Verification items for this drawing (mm, ordinates from the low corner). Round coordinates to 2 decimals unless told otherwise and drop trailing zeros. Write each loop counter-clockwise with the first axis right and the second up, starting at its lowest first coordinate (ties: lowest second). Pieces come first, ordered by that corner, then holes. Notation, with made-up numbers: (-9, -16.75) -> (50, -16.75) arc R6 ccw to (50, -9.75) -> close; hole circle Ø10 at (44, -6.75). An arc over 180 degrees is marked (long way). Put each result on its own line as item: value. Start each with the question number.
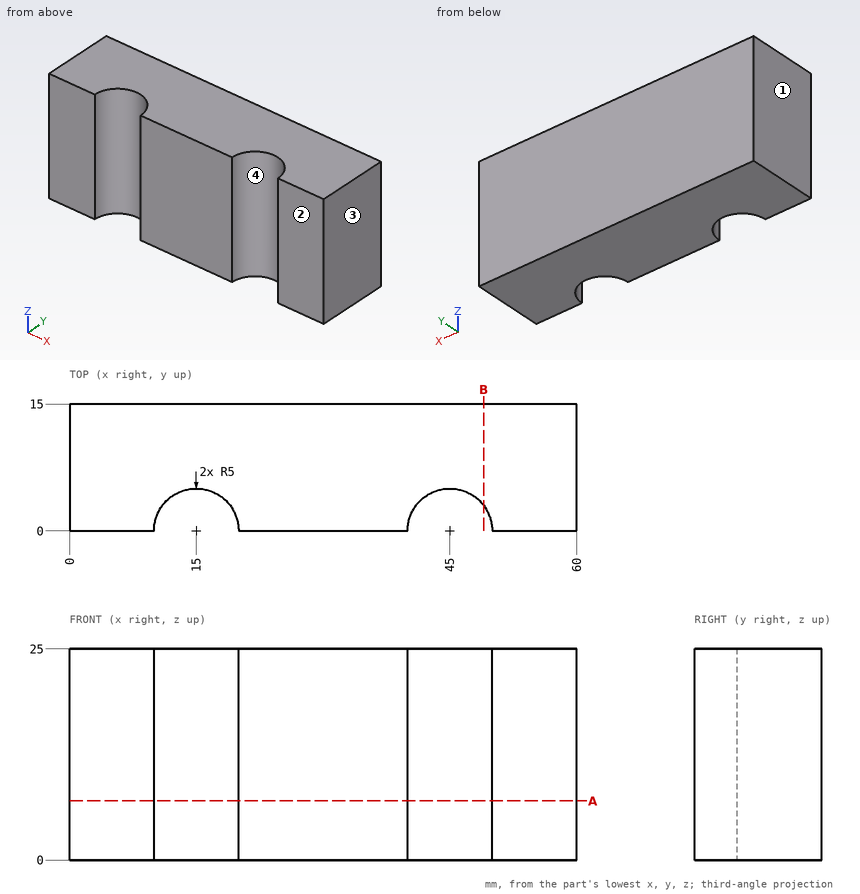
1. Draft check along X on the marked faces 1, 2, 3 and 4. Enter one of: released by +X, released by -X, zero draft, split by the parting line, or undercut.
2. Section check A-A, the plane z = 7. Enter the section's corners in (x, y), then the cut area to 3 significant figures.
3. Section check B-B, the plane x = 49. Enter the section's corners in (y, z), then the cut area to 3 significant figures.
4. Material ranges on L1, parallel to X at y = 2.25, z = 10.5; L2, parallel to X at y = 2.5, z = 9.25; L3, parallel to Y at x = 46, z = 8, recorded low to high. Write a range as [from, to].
Reply:
1. face 1: released by -X
1. face 2: zero draft
1. face 3: released by +X
1. face 4: undercut
2. outline: (0, 0) -> (10, 0) arc R5 cw to (20, 0) -> (40, 0) arc R5 cw to (50, 0) -> (60, 0) -> (60, 15) -> (0, 15) -> close
2. area: 821 mm2
3. outline: (3, 0) -> (15, 0) -> (15, 25) -> (3, 25) -> close
3. area: 300 mm2
4. L1: x = [0, 10.53], [19.47, 40.53], [49.47, 60]
4. L2: x = [0, 10.67], [19.33, 40.67], [49.33, 60]
4. L3: y = [4.9, 15]
